from build123d import *

# Parameters (mm, degrees)
SKETCH_1_W          = 240
SKETCH_1_H          = 160
EXTRUDE_1_DEPTH     = 20
SKETCH_2_R          = 5
CUT_EXTRUDE_1_DEPTH = 20


with BuildPart() as part:
    # 草图1 → 凸台-拉伸1 (new body)
    with BuildSketch(Plane(origin=(0, 0, 0), x_dir=(1, 0, 0), z_dir=(0, 1, 0))):
        Rectangle(SKETCH_1_W, SKETCH_1_H)
    extrude(amount=-EXTRUDE_1_DEPTH)

    # 草图2 → 切除-拉伸1 (cut)
    with BuildSketch(Plane(origin=(0, 0, 0), x_dir=(1, 0, 0), z_dir=(0, 1, 0))):
        with Locations(Location((90, 60, 0), (0, 0, 270))):
            Circle(SKETCH_2_R)
        with Locations(Location((-90, 60, 0), (0, 0, 270))):
            Circle(SKETCH_2_R)
        with Locations(Location((90, -60, 0), (0, 0, 270))):
            Circle(SKETCH_2_R)
        with Locations(Location((-90, -60, 0), (0, 0, 270))):
            Circle(SKETCH_2_R)
    extrude(amount=-CUT_EXTRUDE_1_DEPTH, mode=Mode.SUBTRACT)


solid = part.part
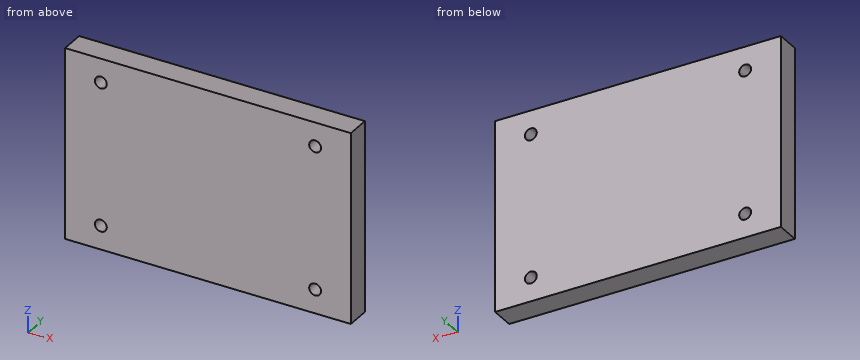
Design review of the part built by this model. Coordinates are the model's own, in mm. Round coordinates to 2 decimals unless told otherwise and drop trailing zeros. Write each loop counter-clockwise with the first axis right and the second up, starting at its lowest first coordinate (ties: lowest second). Pieces come first, ordered by that corner, then holes. Notation, with made-up numbers: (50.5, -29) -> (57.5, -29) arc R22 cw to (57.5, -1) -> close; hole circle Ø11 at (77, 18.25). An arc over 180 degrees is marked (long way). One line per item, written item: value. Start each with the question number.
Q1. To check wall thickness, follow probe 1 along X at (y, z) = (-10.75, -60); probe 2 along X at (y, z) = (-12, 59). State the ranges of each line that lie inside material, in increasing order.
Q2. Add section B-B (x = 90). Give the boundary of the cut face in (y, z), then the cut area to 3 significant figures.
Q3. Add section A-A (z = -60). Give the boundary of the cut face in (x, y), then the cut area to 3 significant figures.
Response:
1. probe 1: x = -120 to -95, -85 to 85, 95 to 120
1. probe 2: x = -120 to -94.9, -85.1 to 85.1, 94.9 to 120
2. outline: (-20, -80) -> (0, -80) -> (0, -65) -> (-20, -65) -> close; (-20, -55) -> (0, -55) -> (0, 55) -> (-20, 55) -> close; (-20, 65) -> (0, 65) -> (0, 80) -> (-20, 80) -> close
2. area: 2,800 mm^2
3. outline: (-120, -20) -> (-95, -20) -> (-95, 0) -> (-120, 0) -> close; (-85, -20) -> (85, -20) -> (85, 0) -> (-85, 0) -> close; (95, -20) -> (120, -20) -> (120, 0) -> (95, 0) -> close
3. area: 4,400 mm^2
